Here's how the part is built. I have some questions about the finished solid (model axes, mm). Round coordinates to 2 decimals unless told otherwise and drop trailing zeros. Order: outer loops, then holes, each group sorted by start corner. A loop starts at its lowest first (then second) coordinate and runs counter-clockwise, first axis right, second up. Notation, with made-up numbers: (-0.5, 62.25) - (18.5, 62.25) arc R29 ccw to (18.5, 86.25) - close; hole circle Ø10 at (54, 55). An arc over 180 degrees is marked (long way). One line per item, written item: value.
from build123d import *

# Parameters (mm, degrees)
SKETCH_1_W      = 24
SKETCH_1_H      = 140
SKETCH_1_R      = 1.5
SKETCH_1_R_2    = 3
EXTRUDE_1_DEPTH = 1.5


with BuildPart() as part:
    # 草图1 → 凸台-拉伸1 (new body)
    with BuildSketch(Plane.XY):
        Rectangle(SKETCH_1_W, SKETCH_1_H)
        with Locations((0, 20)):
            Circle(SKETCH_1_R, mode=Mode.SUBTRACT)
        with Locations((0, -60)):
            Circle(SKETCH_1_R, mode=Mode.SUBTRACT)
        with Locations(Location((0, 60, 0), (0, 0, 180))):
            Circle(SKETCH_1_R, mode=Mode.SUBTRACT)
        with Locations((-9, -11)):
            Circle(SKETCH_1_R, mode=Mode.SUBTRACT)
        with Locations((9, -11)):
            Circle(SKETCH_1_R, mode=Mode.SUBTRACT)
        with Locations((9, -44)):
            Circle(SKETCH_1_R, mode=Mode.SUBTRACT)
        with Locations((-9, -44)):
            Circle(SKETCH_1_R, mode=Mode.SUBTRACT)
        with Locations((0, -20)):
            Circle(SKETCH_1_R_2, mode=Mode.SUBTRACT)
    extrude(amount=EXTRUDE_1_DEPTH)


solid = part.part
Q1. Will these pins go through, and if not, where does the flat tip stop? pin 1 (3.5 mm diameter, centred on x = 0, y = 20, fed in from +Z); pin 2 (2.5 mm diameter, centred on x = 0, y = -60, fed in from -Z).
Results list:
pin 1: z = 1.5
pin 2: through
Q2. If we section it at C-C, the plane y = 60: Please give me the cut outline in (x, z), then the cut area to 3 significant figures.
Results list:
outline: (-12, 0) - (-1.5, 0) - (-1.5, 1.5) - (-12, 1.5) - close; (1.5, 0) - (12, 0) - (12, 1.5) - (1.5, 1.5) - close
area: 31.5 mm²
Q3. We'd pull the mould along Y, two halves only. Please class faces 1 (the flat face through (0, 1, 1.5)), 2 (the cylindrical face through (8.675, -45.464, 0.74)): released by +Y, released by -Y, zero draft, split by the parting line, or undercut.
Results list:
face 1: zero draft
face 2: undercut
Q4. If we section it at A-A, the plane y = -44: Please give me the cut outline in (x, z), then the cut area to 3 significant figures.
Results list:
outline: (-12, 0) - (-10.5, 0) - (-10.5, 1.5) - (-12, 1.5) - close; (-7.5, 0) - (7.5, 0) - (7.5, 1.5) - (-7.5, 1.5) - close; (10.5, 0) - (12, 0) - (12, 1.5) - (10.5, 1.5) - close
area: 27.0 mm²
Q5. If we section it at B-B, the plane x = 0: Please give me the cut outline in (y, z).
Results list:
outline: (-70, 0) - (-61.5, 0) - (-61.5, 1.5) - (-70, 1.5) - close; (-58.5, 0) - (-23, 0) - (-23, 1.5) - (-58.5, 1.5) - close; (-17, 0) - (18.5, 0) - (18.5, 1.5) - (-17, 1.5) - close; (21.5, 0) - (58.5, 0) - (58.5, 1.5) - (21.5, 1.5) - close; (61.5, 0) - (70, 0) - (70, 1.5) - (61.5, 1.5) - close
Q6. If I drill on line 1 along Y through (x, z) = (9, 1.15); line 2 along Y through (x, z) = (0, 0.6); line 3 along Y through (x, z) = (-1.25, 0.85), over which ranges is the centre line in solid material (lowest first)?
Results list:
line 1: -70 to -45.5, -42.5 to -12.5, -9.5 to 70
line 2: -70 to -61.5, -58.5 to -23, -17 to 18.5, 21.5 to 58.5, 61.5 to 70
line 3: -70 to -60.83, -59.17 to -22.73, -17.27 to 19.17, 20.83 to 59.17, 60.83 to 70
Q7. If we section it at D-D, the plane z = 1.25: Give the number of separate pieces and of enclosed holes in the cut face, then the cut area to 3 significant figures.
Results list:
separate pieces: 1
enclosed holes: 8
area: 3,280 mm²
